Autodesk Inventor part; units mm, degrees
ref_plane "YZ Plane" through (0, 0, 0) normal (1, 0, 0) x (0, 1, 0)
ref_plane "XZ Plane" through (0, 0, 0) normal (0, 1, 0) x (-1, 0, 0)
ref_plane "XY Plane" through (0, 0, 0) normal (0, 0, 1) x (1, 0, 0)
sketch "Sketch1" plane through (0, 0, 0) normal (0, 1, 0) x (-1, 0, 0)
  line L0 (0, 0) -> (297, 0)
  line L1 (297, 0) -> (297, -357)
  line L2 (297, -357) -> (0, -357)
  line L3 (0, -357) -> (0, 0)
  line L4 (-19, 19) -> (316, 19)
  line L5 (316, 19) -> (316, -376)
  line L6 (316, -376) -> (-19, -376)
  line L7 (-19, -376) -> (-19, 19)
  dimension "d2" = 19
  dimension "d3" = 19
  dimension "d4" = 19
  dimension "d5" = 19
  dimension "d6" = 395
  dimension "d7" = 335
extrude "Extrusion1" add sketch "Sketch1" along normal mid plane 19
sketch "Sketch3" plane through (0, 9.5, 0) normal (0, 1, 0) x (1, 0, 0)
  line L0 (-316, 376) -> (-316, -19)
  line L1 (-316, 276) -> (-297, 276)
  line L2 (-297, 276) -> (-297, 257)
  line L3 (-297, 257) -> (-316, 257)
  line L4 (-316, 257) -> (-316, 276)
  line L5 (0, 357) -> (0, 0)
  line L6 (19, 376) -> (19, -19)
  line L7 (0, 276) -> (19, 276)
  line L8 (19, 276) -> (19, 257)
  line L9 (19, 257) -> (0, 257)
  line L10 (0, 257) -> (0, 276)
  line L11 (19, 376) -> (-316, 376)
  dimension "d26" = 19
  dimension "d27" = 19
  dimension "d28" = 100
extrude "Extrusion2" add sketch "Sketch3" along normal blind 460
sketch "Sketch4" plane through (-297, -9.5, 0) normal (1, 0, 0) x (0, 0, -1)
  line L0 (257, 19) -> (257, 479)
  line L1 (276, 19) -> (276, 479)
  line L2 (257, 479) -> (276, 479)
  line L3 (276, 479) -> (276, 460)
  line L4 (276, 460) -> (257, 460)
  line L5 (257, 460) -> (257, 479)
  point P0 (0, 9.5)
  dimension "d31" = 19
extrude "Extrusion3" add sketch "Sketch4" along normal blind 316
sketch "Sketch5" plane through (19, 469.5, -276) normal (0, 0, -1) x (-1, 0, 0)
  circle A0 centre (9.5, -100) radius 4
  circle A1 centre (325.5, -100) radius 4
  circle A2 centre (9.5, -360) radius 4
  circle A3 centre (325.5, -360) radius 4
  line L0 (335, -460) -> (335, 0)
  line L1 (0, 0) -> (335, 0)
  line L2 (19, -460) -> (19, -19)
  line L3 (0, -460) -> (335, -460)
  line L4 (0, -460) -> (0, 0)
  point P0 (19, -469.5)
  dimension "d34" = 8
  dimension "d35" = 8
  dimension "d36" = 8
  dimension "d37" = 8
  dimension "d38" = 9.5
  dimension "d39" = 100
  dimension "d40" = 100
  dimension "d41" = 9.5
  dimension "d42" = 9.5
  dimension "d43" = 100
  dimension "d44" = 100
  dimension "d45" = 9.5
extrude "Extrusion4" cut sketch "Sketch5" against normal blind 19 contours A0 | A1 | A2 | A3
sketch "Sketch6" plane through (0, 9.5, 0) normal (0, 1, 0) x (1, 0, 0)
  line L0 (19, 376) -> (19, -19)
  line L1 (-316, 257) -> (19, 257)
  line L2 (19, 257) -> (19, 238)
  line L3 (19, 238) -> (-316, 238)
  line L4 (-316, 238) -> (-316, 257)
  line L5 (19, 376) -> (-316, 376)
  point P0 (0, 0)
  dimension "d48" = 19
  dimension "d49" = 335
  dimension "d51" = 119
extrude "Extrusion5" add sketch "Sketch6" along normal blind 19
sketch "Sketch7" plane through (0, 28.5, 0) normal (0, 1, 0) x (1, 0, 0)
  circle A0 centre (-306.5, 247.5) radius 4
  circle A1 centre (9.5, 247.5) radius 4
  line L0 (19, 238) -> (19, 257)
  line L1 (-316, 238) -> (19, 238)
  line L2 (-316, 257) -> (-316, 238)
  point P0 (0, 0)
  dimension "d54" = 8
  dimension "d55" = 8
  dimension "d56" = 9.5
  dimension "d57" = 9.5
  dimension "d58" = 9.5
  dimension "d59" = 9.5
extrude "Extrusion6" cut sketch "Sketch7" against normal blind 39
sketch "Sketch8" plane through (19, 469.5, -276) normal (0, 0, -1) x (-1, 0, 0)
  line L0 (335, -460) -> (0, -460)
  line L1 (335, -460) -> (335, 0)
  line L2 (0, -460) -> (335, -460)
  line L3 (335, -460) -> (335, 0)
  line L4 (335, 0) -> (0, 0)
  line L5 (0, 0) -> (0, -460)
  point P0 (19, -469.5)
extrude "Extrusion7" add sketch "Sketch8" along normal blind 4
properties part number "Test stand v1.2"
Geometry check sheet. Reference: the model listing, model coordinates, mm. A direction names the side the tool comes from. Give positions to 0.01 mm unless a question says otherwise; leave off trailing zeros. Loops run counter-clockwise (first coordinate to the right, second up) from the corner with the lowest first, then second, coordinate; pieces in that order, holes last. Notation, with made-up numbers: M 35,-1 L 42,-1 A24 cw 42,34 Z; hole C -16,66 d8. An arc over 180 degrees is marked long. Write item = value, one per line. Start each with the question number.
1. Section check B-B, the plane x = -237.5. Enter the section's corners in (y, z).
2. Draft check along X on faces 4 (the face through (-297, 151, -270)), 5 (the face through (19, 160, -265)), 6 (the face through (-151, 469.5, -268)), 7 (the face through (-316, 158, -265)). Enter one of: +X half, -X half, draft (parallel to the pull), parting line (faces both ways), or undercut.
3. Thickness scan on probe 1 along X at (y, z) = (369.5, -261.5); probe 2 along Y at (x, z) = (-306, -268); probe 3 along Z at (x, y) = (-264.5, 19.5). Record the ranges inside material, lowest first.
4. Go/stop test with flat-tipped pins: P1, Ø1, axis at x = -18, y = 338, coming from the +Z side; P2, Ø3, axis at x = -136, z = -278.5, coming from the -Y side; P3, Ø13, axis at x = 9.5, y = 369.5, coming from the +Z side. Record where each tip stops, or that it passes through.
5. Tool access check on faces 1 (the face through (-151, 9.5, -248)), 2 (the face through (-110, 9.5, 5)), 3 (the face through (-146, 0, 0)). Record the directions out of +Z, -Z, +X, -X, +Y, -Y that give a thin tool (end or side, any length) a straight path to the whole face; none if there is none.
6. Section check A-A, the plane z = -313. Enter the section's corners in (x, y).
7. Section check C-C, the plane y = 309.5. Enter the section's corners in (x, z).
Values follow:
q1.outline = M -9.5,-376 L 9.5,-376 L 9.5,-357 L -9.5,-357 Z; M -9.5,0 L 9.5,0 L 9.5,19 L -9.5,19 Z; M 9.5,-280 L 469.5,-280 L 469.5,-257 L 450.5,-257 L 450.5,-276 L 9.5,-276 Z; M 9.5,-257 L 28.5,-257 L 28.5,-238 L 9.5,-238 Z
q2.face_4 = undercut
q2.face_5 = +X half
q2.face_6 = draft
q2.face_7 = -X half
q3.probe_1 = -316 to -310.5, -302.5 to -297, 0 to 5.5, 13.5 to 19
q3.probe_2 = -9.5 to 105.53, 113.47 to 365.53, 373.47 to 469.5
q3.probe_3 = -280 to -276, -257 to -238
q4.P1 = -276
q4.P2 = 9.5
q4.P3 = -257
q5.face_1 = -Y
q5.face_2 = +Z, +X, -X, +Y
q5.face_3 = +Y, -Y
q6.outline = M -316,-9.5 L -297,-9.5 L -297,9.5 L -316,9.5 Z; M 0,-9.5 L 19,-9.5 L 19,9.5 L 0,9.5 Z
q7.outline = M -316,-280 L 19,-280 L 19,-257 L 0,-257 L 0,-276 L -297,-276 L -297,-257 L -316,-257 Z
